```python
from build123d import *

# Parameters (mm, degrees)
F0_R     = 35.9798684942
F1_DEPTH = 150
F2_T     = -2.5
F4_W     = 21.6136686504
F4_H     = 64.6223351359
F5_DEPTH = 150


with BuildPart() as f1:
    # F0 (on Top) → F1 (new body)
    with BuildSketch(Plane.XY):
        Circle(F0_R)
    extrude(amount=F1_DEPTH)

    # F2
    f2_openings = [f1.faces().sort_by_distance(p)[0] for p in [
        (0, 0, 150),
    ]]
    offset(amount=F2_T, openings=f2_openings)

    # F4 (on face) → F5 (cut)
    with BuildSketch(Plane(origin=(35.9798684942, 0, 0), x_dir=(0, -1, 0), z_dir=(-1, 0, 0))):
        with Locations((10.8068343252, 42.1714968979)):
            Rectangle(F4_W, F4_H)
        with Locations((-10.8068343252, 42.1714968979)):
            Rectangle(F4_W, F4_H)
    extrude(amount=F5_DEPTH, mode=Mode.SUBTRACT)


solid = f1.part
```
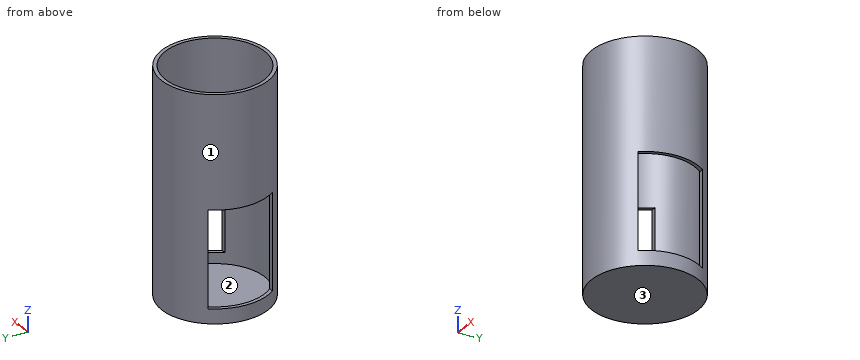
Input: part model. Units: mm. Frame: model coordinates. Face numbers are marked on the shaded views. Coordinates: 2 decimals unless noted, no trailing zeros. Write each loop counter-clockwise with the first axis right and the second up, starting at its lowest first coordinate (ties: lowest second). Pieces come first, ordered by that corner, then holes. Notation, with made-up numbers: (54, -19.75) -> (80, -19.75) arc R26 ccw to (80, 2.25) -> close; hole circle Ø4 at (-33.75, -23.75). An arc over 180 degrees is marked (long way). Answer as a JSON object with one key per item and string values.
1. Section A-A on z = 30. Return the cut outline in (x, y), then the cut area to 3 significant figures.
Result set:
{"outline": "(-28.76, -21.61) arc R35.98 ccw to (28.76, -21.61) -> (25.57, -21.61) arc R33.48 cw to (-25.57, -21.61) -> close; (-28.76, 21.61) -> (-25.57, 21.61) arc R33.48 cw to (25.57, 21.61) -> (28.76, 21.61) arc R35.98 ccw to start", "area": "312 mm2"}
2. Mould query, pull axis Y, two halves, no side actions, for the marked faces 1, 2 and 3. Classes: released by +Y, released by -Y, zero draft, split by the parting line, or undercut.
Result set:
{"face 1": "split by the parting line", "face 2": "undercut", "face 3": "zero draft"}
3. Section C-C on x = 0. Return the cut outline in (y, z), then the cut area to 3 significant figures.
Result set:
{"outline": "(-35.98, 0) -> (35.98, 0) -> (35.98, 150) -> (33.48, 150) -> (33.48, 2.5) -> (-33.48, 2.5) -> (-33.48, 150) -> (-35.98, 150) -> close", "area": "917 mm2"}
4. Material intervals for line 1 (Z direction, x = -32, y = 15); line 2 (Y direction, x = 0, z = 112), sorted ascending. Write a range as from..to.
Result set:
{"line 1": "z = 0..9.86, 74.48..150", "line 2": "y = -35.98..-33.48, 33.48..35.98"}
5. Section B-B on y = 0. Return the cut outline in (x, z), then the cut area to 3 significant figures.
Result set:
{"outline": "(-35.98, 0) -> (35.98, 0) -> (35.98, 9.86) -> (33.48, 9.86) -> (33.48, 2.5) -> (-33.48, 2.5) -> (-33.48, 9.86) -> (-35.98, 9.86) -> close; (-35.98, 74.48) -> (-33.48, 74.48) -> (-33.48, 150) -> (-35.98, 150) -> close; (33.48, 74.48) -> (35.98, 74.48) -> (35.98, 150) -> (33.48, 150) -> close", "area": "594 mm2"}
6. Section D-D on z = 137. Return the cut outline in (x, y).
Result set:
{"outline": "circle Ø71.96 at (0, 0); hole circle Ø66.96 at (0, 0)"}
7. First-contact query: P1, Ø1, axis at x = -17.5, y = -20, coming from the +Z side; P2, Ø1, axis at x = 27, z = 42, coming from the -Y side; P3, Ø2, axis at x = 10.5, z = 111.5, coming from the -Y side. Flat tips, straight axial feed; report the tip coordinate or a pass-through.
Result set:
{"P1": "stops at z = 2.5", "P2": "stops at y = -24.34", "P3": "stops at y = -34.7"}
